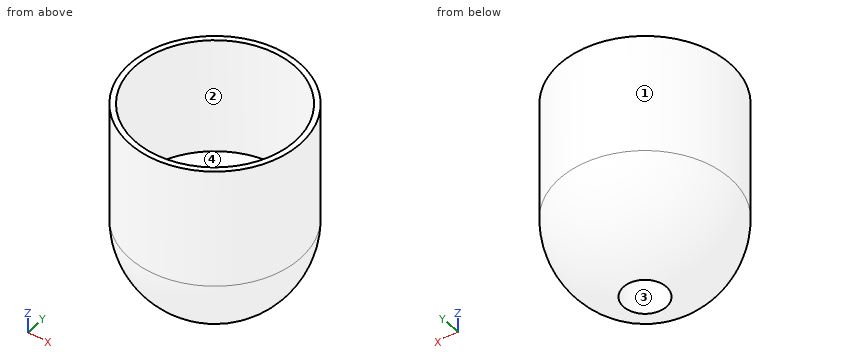
from build123d import *

# Parameters (mm, degrees)
SKETCH1_R           = 22.62
BOSS_EXTRUDE1_DEPTH = 32
SKETCH3_R           = 5.673095137
CUT_EXTRUDE1_DEPTH  = 76
SKETCH5_R           = 21.203687462
CUT_EXTRUDE2_DEPTH  = 31


with BuildPart() as part:
    # Sketch1 → Boss-Extrude1 (new body)
    with BuildSketch(Plane.XY):
        Circle(SKETCH1_R)
    extrude(amount=BOSS_EXTRUDE1_DEPTH)

    # Sketch2 one side → Revolve1 (revolve)
    with BuildSketch(Plane(origin=(0, 0, 0), x_dir=(-1, 0, 0), z_dir=(0, 0, -1))):
        with BuildLine():
            ThreePointArc((0, 22.62), (-22.62, 0), (0, -22.62))
            Line((0, -22.62), (0, 0))
            Line((0, 0), (0, 22.62))
        make_face()
    revolve(axis=Axis((0, 0, 0), (0, 1, 0)))

    # Sketch3 → Cut-Extrude1 (cut)
    with BuildSketch(Plane.XY.offset(32)):
        Circle(SKETCH3_R)
    extrude(amount=-CUT_EXTRUDE1_DEPTH, mode=Mode.SUBTRACT)

    # Sketch5 → Cut-Extrude2 (cut)
    with BuildSketch(Plane.XY.offset(32)):
        Circle(SKETCH5_R)
    extrude(amount=-CUT_EXTRUDE2_DEPTH, mode=Mode.SUBTRACT)


solid = part.part
Could you check a few things on this model? Use its own coordinates, in mm. Face numbers are marked on the shaded views. A direction names the side the tool comes from. Round coordinates to 2 decimals unless told otherwise and drop trailing zeros. Write each loop counter-clockwise with the first axis right and the second up, starting at its lowest first coordinate (ties: lowest second). Pieces come first, ordered by that corner, then holes. Notation, with made-up numbers: (77.5, 74) - (110.5, 74) arc R23 ccw to (110.5, 110) - close; hole circle Ø11 at (69.5, -32.5). An arc over 180 degrees is marked (long way). Use a Markdown table: item, result.
Q1. For pin 1 (5 mm diameter, centred on x = 0.5, y = -9, fed in from -Z); pin 2 (5 mm diameter, centred on y = 8, z = -13, fed in from +X); pin 3 (12 mm diameter, centred on x = -4, y = 10.5, fed in from +Z), each with a flat end and sliding along its axis, tell me the tip position at first contact or that it passes through.
Output values:
| item | result |
|---|---|
| pin 1 | z = -21.66 |
| pin 2 | x = 18.67 |
| pin 3 | z = 1 |
Q2. Thinking about a two-plate mould opening in Y: for the marked faces 1 and 2, which applies, released by +Y, released by -Y, zero draft, split by the parting line, or undercut?
Output values:
| item | result |
|---|---|
| face 1 | split by the parting line |
| face 2 | undercut |
Q3. I want a section at D-D (z = -5.5). List the corners of the cut face in (x, y) for me, plus the area to 3 significant figures.
Output values:
| item | result |
|---|---|
| outline | circle Ø43.88 at (0, 0); hole circle Ø11.35 at (0, 0) |
| area | 1,410 mm2 |
Q4. Please list where these lines run through material, in increasing order: L1, parallel to Y at x = 0, z = 21; L2, parallel to X at y = 3.5, z = 29.5; L3, parallel to X at y = 0, z = -10.
Output values:
| item | result |
|---|---|
| L1 | -22.62 to -21.2, 21.2 to 22.62 |
| L2 | -22.35 to -20.91, 20.91 to 22.35 |
| L3 | -20.29 to -5.67, 5.67 to 20.29 |
Q5. I want a section at A-A (x = 0). List the corners of the cut face in (y, z) for me.
Output values:
| item | result |
|---|---|
| outline | (-22.62, 0) arc R22.62 ccw to (-5.67, -21.9) - (-5.67, 1) - (-21.2, 1) - (-21.2, 32) - (-22.62, 32) - close; (5.67, -21.9) arc R22.62 ccw to (22.62, 0) - (22.62, 32) - (21.2, 32) - (21.2, 1) - (5.67, 1) - close |
Q6. For the marked faces 3 and 4, which set-ups out of +Z, -Z, +X, -X, +Y, -Y let a thin tool reach every point of the face, with its end or its side?
Output values:
| item | result |
|---|---|
| face 3 | +Z, -Z |
| face 4 | +Z |
Q7. I want a section at C-C (x = -13). List the corners of the cut face in (y, z) for me.
Output values:
| item | result |
|---|---|
| outline | (-18.51, 0) arc R18.51 ccw to (18.51, 0) - (18.51, 32) - (16.75, 32) - (16.75, 1) - (-16.75, 1) - (-16.75, 32) - (-18.51, 32) - close |
